The listing builds one solid part. Answer for the finished solid, in the listing's coordinates (mm). Face numbers are marked on the shaded views. A direction names the side the tool comes from. Coordinates: 2 decimals unless noted, no trailing zeros. Loops run counter-clockwise (first coordinate to the right, second up) from the corner with the lowest first, then second, coordinate; pieces in that order, holes last. Notation, with made-up numbers: (86, 57.25) - (132, 57.25) arc R23 cw to (132, 83.25) - close; hole circle Ø1 at (75, -22). An arc over 180 degrees is marked (long way). One line per question, with ' | ' between items.
from build123d import *

# Parameters (mm, degrees)
SKETCH_W     = 100
SKETCH_H     = 50
PAD_DEPTH    = 5
SKETCH001_R  = 5
POCKET_DEPTH = 5
SKETCH002_W  = 100
SKETCH002_H  = 5
PAD001_DEPTH = 25
FILLET_R     = 20
FILLET001_R  = 10
FILLET002_R  = 5


with BuildPart() as part:
    # Sketch → Pad (new body)
    with BuildSketch(Plane.XY):
        Rectangle(SKETCH_W, SKETCH_H)
    extrude(amount=PAD_DEPTH)

    # Sketch001 (on Face6 of Pad) → Pocket (cut)
    with BuildSketch(Plane.XY.offset(5)):
        with Locations((40, 15)):
            Circle(SKETCH001_R)
        with Locations((40, -15)):
            Circle(SKETCH001_R)
        with Locations((-40, 15)):
            Circle(SKETCH001_R)
        with Locations((-40, -15)):
            Circle(SKETCH001_R)
    extrude(amount=-POCKET_DEPTH, mode=Mode.SUBTRACT)

    # Sketch002 (on Face5 of Pocket) → Pad001 (join)
    with BuildSketch(Plane.XY.offset(5)):
        Rectangle(SKETCH002_W, SKETCH002_H)
    extrude(amount=PAD001_DEPTH)

    # Fillet
    fillet_edges = [part.edges().sort_by_distance(p)[0] for p in [
        (50, 0, 30),
        (-50, 0, 30),
    ]]
    fillet(fillet_edges, radius=FILLET_R)

    # Fillet001
    fillet001_edges = [part.edges().sort_by_distance(p)[0] for p in [
        (50, -25, 2.5),
        (-50, -25, 2.5),
        (-50, 25, 2.5),
        (50, 25, 2.5),
    ]]
    fillet(fillet001_edges, radius=FILLET001_R)

    # Fillet002
    fillet002_edges = [part.edges().sort_by_distance(p)[0] for p in [
        (0, -2.5, 5),
        (0, 2.5, 5),
    ]]
    fillet(fillet002_edges, radius=FILLET002_R)


solid = part.part
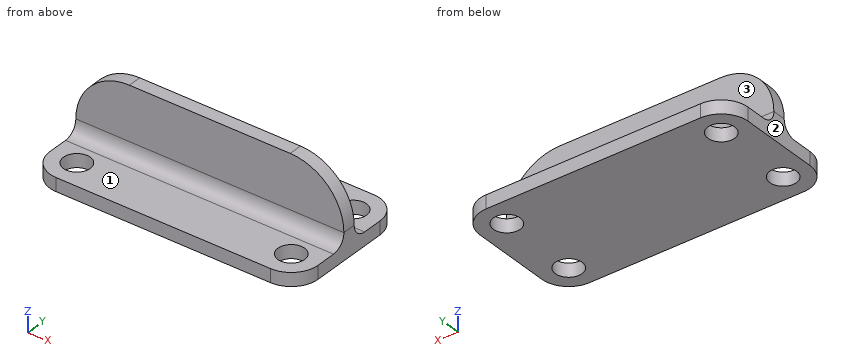
Item 1: Which of the six approach directions +Z, -Z, +X, -X, +Y, -Y give full straight-line access (tool end or side, diameter ignored) to the marked faces 1, 2 and 3?
Taken from the geometry:
face 1: +Z, +X, -X, -Y | face 2: +Z, -Z, -X, +Y, -Y | face 3: +Z, +X, -X, +Y
Item 2: Find section D-D, the plane z = 17. Write down the section's boundary in (x, y) (3 decimals).
Taken from the geometry:
outline: (-48.735, -2.5) - (48.735, -2.5) - (48.735, 2.5) - (-48.735, 2.5) - close
Item 3: Find the intervals of material crossed by line 1 (Y direction, x = 40, z = 3.45); line 2 (Y direction, x = 43, z = 3); line 3 (Z direction, x = 10.5, y = -21), in increasing order. Write a range as [from, to].
Taken from the geometry:
line 1: y = [-25, -20], [-10, 10], [20, 25] | line 2: y = [-24.54, -19], [-11, 11], [19, 24.54] | line 3: z = [0, 5]
Item 4: Find section A-A, the plane x = 28. Write down the section's boundary in (y, z), plus the area to 3 significant figures.
Taken from the geometry:
outline: (-25, 0) - (25, 0) - (25, 5) - (7.5, 5) arc R5 cw to (2.5, 10) - (2.5, 30) - (-2.5, 30) - (-2.5, 10) arc R5 cw to (-7.5, 5) - (-25, 5) - close | area: 386 mm2
Item 5: Find section B-B, the plane y = -11.5. Write down the section's boundary in (x, z), plus the area to 3 significant figures.
Taken from the geometry:
outline: (-50, 0) - (-43.57, 0) - (-43.57, 5) - (-50, 5) - close; (-36.43, 0) - (36.43, 0) - (36.43, 5) - (-36.43, 5) - close; (43.57, 0) - (50, 0) - (50, 5) - (43.57, 5) - close | area: 429 mm2
Item 6: Each of these flat-tipped pins is pushed along its axis until it touches: pin 1 Ø8 at (x, y) = (-40, 15) entering from -Z; pin 2 Ø1 at (x, z) = (24.5, 7.5) entering from +Y; pin 3 Ø9 at (x, y) = (-5.5, -20) entering from +Z; pin 4 Ø14 at (x, y) = (-4, 12.5) entering from +Z. Where does it stop, or does it pass through?
Taken from the geometry:
pin 1: passes through | pin 2: stops at y = 3.5 | pin 3: stops at z = 5 | pin 4: stops at z = 5.42
Item 7: Find section C-C, the plane y = 3.5. Write down the section's boundary in (x, z), plus the area to 3 significant figures.
Taken from the geometry:
outline: (-50, 0) - (50, 0) - (50, 7) - (-50, 7) - close | area: 700 mm2
